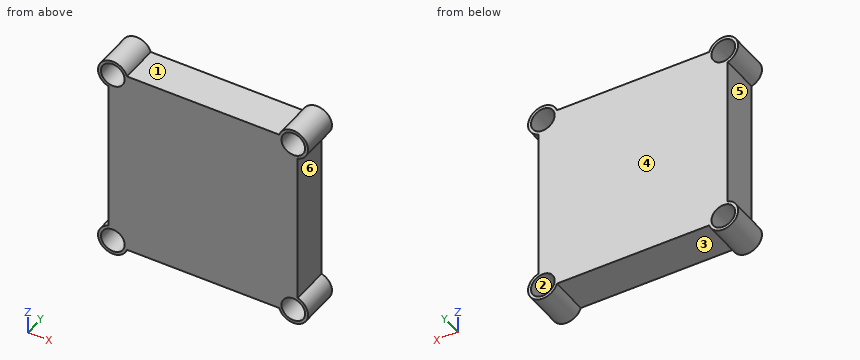
from build123d import *

# Parameters (mm, degrees)
SKETCH1_R           = 2.5
SKETCH1_W           = 32
SKETCH1_H           = 32
BOSS_EXTRUDE1_DEPTH = 6.6
SKETCH2_R           = 2
CUT_EXTRUDE1_DEPTH  = 10


with BuildPart() as part:
    # Sketch1 → Boss-Extrude1 (new body)
    with BuildSketch(Plane(origin=(0, 0, 0), x_dir=(1, 0, 0), z_dir=(0, 1, 0))):
        with Locations((-15.25, 15.25)):
            Circle(SKETCH1_R)
        with Locations((15.25, 15.25)):
            Circle(SKETCH1_R)
        with Locations((-15.25, -15.25)):
            Circle(SKETCH1_R)
        with Locations((15.25, -15.25)):
            Circle(SKETCH1_R)
        Rectangle(SKETCH1_W, SKETCH1_H)
    extrude(amount=BOSS_EXTRUDE1_DEPTH)

    # Sketch2 → Cut-Extrude1 (cut)
    with BuildSketch(Plane(origin=(0, 6.6, 0), x_dir=(1, 0, 0), z_dir=(0, 1, 0))):
        with Locations(Location((-15.25, 15.25, 0), (0, 0, 270))):
            Circle(SKETCH2_R)
        with Locations(Location((15.25, 15.25, 0), (0, 0, 270))):
            Circle(SKETCH2_R)
        with Locations(Location((15.25, -15.25, 0), (0, 0, 270))):
            Circle(SKETCH2_R)
        with Locations(Location((-15.25, -15.25, 0), (0, 0, 270))):
            Circle(SKETCH2_R)
    extrude(amount=-CUT_EXTRUDE1_DEPTH, mode=Mode.SUBTRACT)


solid = part.part
Check sheet for the modelled part. Datum: model origin and axes. Units: mm. Face numbers are marked on the shaded views. A direction names the side the tool comes from. Give positions to 0.01 mm unless a question says otherwise; leave off trailing zeros. Order: outer loops, then holes, each group sorted by start corner. A loop starts at its lowest first (then second) coordinate and runs counter-clockwise, first axis right, second up. Notation, with made-up numbers: (27.5, 84.5) - (65.5, 84.5) arc R18 ccw to (65.5, 96.5) - close; hole circle Ø6 at (-37.5, -32.75). An arc over 180 degrees is marked (long way). Answer as CSV lines item,"result".
1. Mould release check, pull along Z, two halves, no side actions. Record for the marked faces 1, 2 and 3: released by +Z, released by -Z, zero draft, split by the parting line, or undercut.
Result sheet:
face 1,"released by +Z"
face 2,"undercut"
face 3,"released by -Z"
2. Section check A-A (z = -15.25). Record the boundary of the cut face in (x, y).
Result sheet:
outline,"(-17.75, 0) - (-17.25, 0) - (-17.25, 6.6) - (-17.75, 6.6) - close; (-13.25, 0) - (13.25, 0) - (13.25, 6.6) - (-13.25, 6.6) - close; (17.25, 0) - (17.75, 0) - (17.75, 6.6) - (17.25, 6.6) - close"
3. Section check C-C (y = 5). Record the boundary of the cut face in (x, z), then the cut area to 3 significant figures.
Result sheet:
outline,"(-16, -12.87) arc R2.5 ccw (long way) to (-12.87, -16) - (12.87, -16) arc R2.5 ccw (long way) to (16, -12.87) - (16, 12.87) arc R2.5 ccw (long way) to (12.87, 16) - (-12.87, 16) arc R2.5 ccw (long way) to (-16, 12.87) - close; hole circle Ø4 at (-15.25, -15.25); hole circle Ø4 at (-15.25, 15.25); hole circle Ø4 at (15.25, -15.25); hole circle Ø4 at (15.25, 15.25)"
area,"1,020 mm²"
4. Section check B-B (x = 15.25). Record the boundary of the cut face in (y, z).
Result sheet:
outline,"(0, -17.75) - (6.6, -17.75) - (6.6, -17.25) - (0, -17.25) - close; (0, -13.25) - (6.6, -13.25) - (6.6, 13.25) - (0, 13.25) - close; (0, 17.25) - (6.6, 17.25) - (6.6, 17.75) - (0, 17.75) - close"
5. Scan lines: probe 1 along X at (y, z) = (5, 15.25); probe 2 along Z at (x, y) = (14.5, 5.25); probe 3 along X at (y, z) = (2, -6.5). Record each from-to range of solid material in increasing order. Write a range as from..to.
Result sheet:
probe 1,"-17.75..-17.25, -13.25..13.25, 17.25..17.75"
probe 2,"-17.63..-17.1, -13.4..13.4, 17.1..17.63"
probe 3,"-16..16"
6. Tool access check on the marked faces 4, 5 and 6. Record the directions out of +Z, -Z, +X, -X, +Y, -Y that give a thin tool (end or side, any length) a straight path to the whole face; none if there is none.
Result sheet:
face 4,"+Z, -Z, +X, -X, +Y"
face 5,"-X, +Y, -Y"
face 6,"+X, +Y, -Y"
7. Section check D-D (x = 2). Record the boundary of the cut face in (y, z).
Result sheet:
outline,"(0, -16) - (6.6, -16) - (6.6, 16) - (0, 16) - close"
8. Go/stop test with flat-tipped pins: P1, Ø3.5, axis at y = 4, z = 4, coming from the +X side; P2, Ø3.5, axis at x = -0.5, y = 3.5, coming from the +Z side; P3, Ø2, axis at y = 2, z = -2.5, coming from the -X side. Record where each tip stops, or that it passes through.
Result sheet:
P1,"x = 16"
P2,"z = 16"
P3,"x = -16"
